Job drawing, mm, ordinate dimensions from the low corner. One solid piece. A direction names the side the tool comes from. Coordinates: 2 decimals unless noted, no trailing zeros. Order: outer loops, then holes, each group sorted by start corner. A loop starts at its lowest first (then second) coordinate and runs counter-clockwise, first axis right, second up. Notation, with made-up numbers: (-5.5, 27.25) - (23.5, 27.25) arc R18 cw to (23.5, 49.25) - close; hole circle Ø4 at (-10, 24.25). An arc over 180 degrees is marked (long way). Use a Markdown table: item, result. Add a question column.
1) Drop flat-ended pins along their axis: P1, Ø3, axis at x = 11, y = 2.5, coming from the -Z side; P2, Ø2, axis at x = 5.5, y = 7, coming from the +Z side. Give the stop position or say it passes through.
2) Saw through at B-B on z = 3. List the corners of the cut face in (x, y).
3) Tool access for the marked faces 1 and 2: list every direction of +Z, -Z, +X, -X, +Y, -Y with a clear straight run to the whole face (end or side of a thin tool).
4) Saw through at A-A on x = 11. List the corners of the cut face in (y, z), then the cut area to 3 significant figures.
5) Wall check: L1, parallel to Z at x = 16, y = 2.5; L2, parallel to X at y = 18.5, z = 0.75; L3, parallel to Z at x = 7, y = 1.25. Give the ranges that are in metal, low to high. Write a range as [from, to].
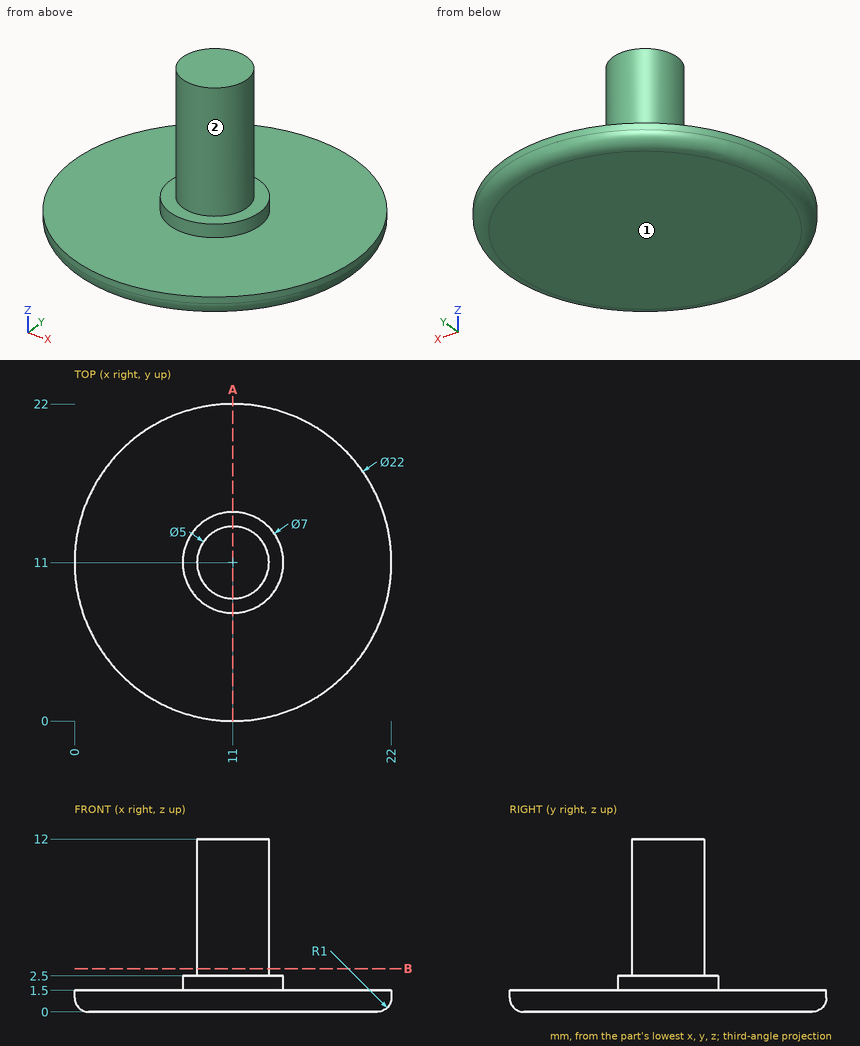
Results are:
| question | item | result |
|---|---|---|
| 1 | P1 | z = 0 |
| 1 | P2 | z = 1.5 |
| 2 | outline | circle Ø5 at (11, 11) |
| 3 | face 1 | -Z, +X, -X, +Y, -Y |
| 3 | face 2 | +Z |
| 4 | outline | (0, 1) arc R1 ccw to (1, 0) - (21, 0) arc R1 ccw to (22, 1) - (22, 1.5) - (14.5, 1.5) - (14.5, 2.5) - (13.5, 2.5) - (13.5, 12) - (8.5, 12) - (8.5, 2.5) - (7.5, 2.5) - (7.5, 1.5) - (0, 1.5) - close |
| 4 | area | 87.1 mm2 |
| 5 | L1 | [0, 1.5] |
| 5 | L2 | [3, 19] |
| 5 | L3 | [0.16, 1.5] |
